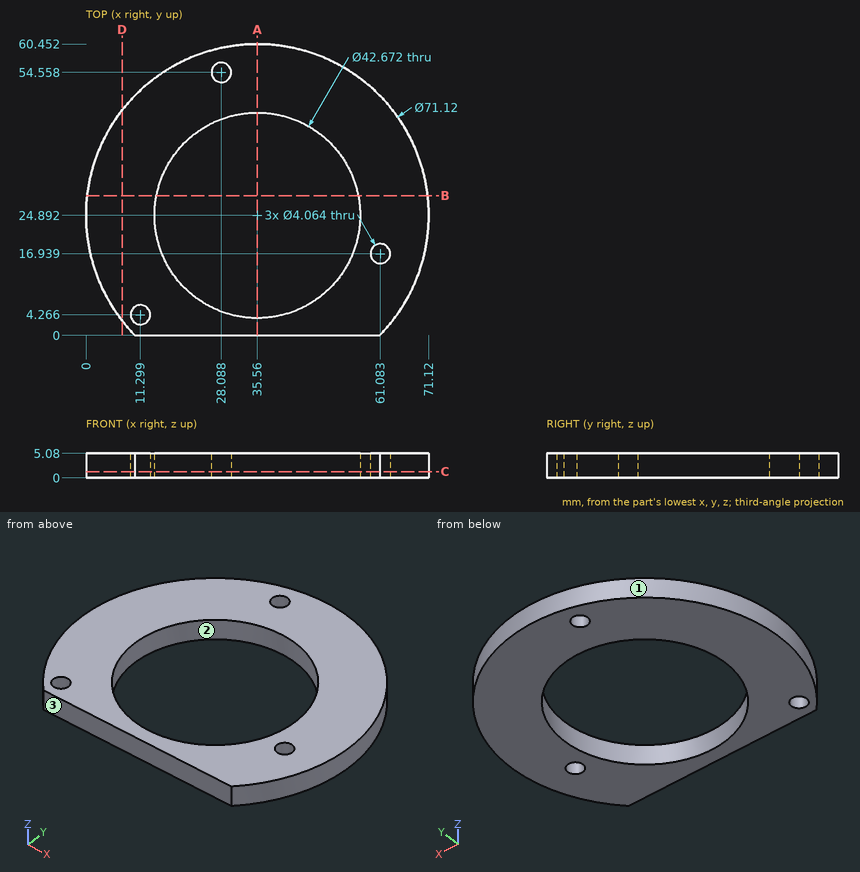
Source: three-view drawing plus pictorial views. Frame: mm from the lowest corner of the part. Round coordinates to 2 decimals unless told otherwise and drop trailing zeros. Loops run counter-clockwise (first coordinate to the right, second up) from the corner with the lowest first, then second, coordinate; pieces in that order, holes last.
1. Section query A-A on x = 35.56. Output: boundary loops of the cut face in (y, z).
2. Contact query for flat-ended pins moving along their axis: pin 1 (1 mm diameter, centred on x = 59.5, z = 2, fed in from +Y); pin 2 (2 mm diameter, centred on y = 51.5, z = 4.5, fed in from +X); pin 3 (3.5 mm diameter, centred on x = 11.3, y = 4.27, fed in from -Z); pin 4 (1.5 mm diameter, centred on y = 40.5, z = 1, fed in from -X). Output: stop coordinate, or through.
3. Ray query, L1, parallel to X at y = 17.5, z = 4.1 (1 decimal); L2, parallel to Y at x = 28, z = 2.7 (1 decimal); L3, parallel to Y at x = 24.5, z = 3.1 (1 decimal). Return the intervals inside material, ascending.
4. Section query C-C on z = 1.25. Output: boundary loops of the cut face in (x, y) (1 decimal).
5. Section query B-B on y = 29. Output: boundary loops of the cut face in (x, z).
6. Section query D-D on x = 7.5. Output: boundary loops of the cut face in (y, z) (1 decimal), and give its area (3 significant figures).
7. Mould query, pull axis Y, two halves, no side actions, for the marked faces 1, 2 and 3. Classes: released by +Y, released by -Y, zero draft, split by the parting line, or undercut.
Answers below:
1. outline: (0, 0) - (3.56, 0) - (3.56, 5.08) - (0, 5.08) - close; (46.23, 0) - (60.45, 0) - (60.45, 5.08) - (46.23, 5.08) - close
2. pin 1: stops at y = 51.63
2. pin 2: stops at x = 60.23
2. pin 3: passes through
2. pin 4: stops at x = 3.25
3. L1: x = 0.8 to 15.5, 55.6 to 59.1, 63 to 70.3
3. L2: y = 0 to 4.9, 44.8 to 52.5, 56.6 to 59.6
3. L3: y = 0 to 6.6, 43.1 to 58.7
4. outline: (10.2, 0) - (61, 0) arc R35.6 ccw (long way) to start; hole circle Ø4.1 at (11.3, 4.3); hole circle Ø42.7 at (35.6, 24.9); hole circle Ø4.1 at (28.1, 54.6); hole circle Ø4.1 at (61.1, 16.9)
5. outline: (0.24, 0) - (14.62, 0) - (14.62, 5.08) - (0.24, 5.08) - close; (56.5, 0) - (70.88, 0) - (70.88, 5.08) - (56.5, 5.08) - close
6. outline: (3, 0) - (46.7, 0) - (46.7, 5.1) - (3, 5.1) - close
6. area: 222 mm2
7. face 1: split by the parting line
7. face 2: undercut
7. face 3: released by -Y
